```python
from build123d import *

# Parameters (mm, degrees)
SKETCH1_W           = 76.454
SKETCH1_H           = 69.596
BOSS_EXTRUDE1_DEPTH = 7.62
SKETCH2_W           = 71.374
SKETCH2_H           = 64.516
CUT_EXTRUDE1_DEPTH  = 5.08
SKETCH4_W           = 5.08
SKETCH4_H           = 5.08
BOSS_EXTRUDE2_DEPTH = 8.7884
CUT_EXTRUDE2_DEPTH  = 5.08
SKETCH6_W           = 2.54
SKETCH6_H           = 2.54
BOSS_EXTRUDE3_DEPTH = 29.21
SKETCH7_W           = 76.454
SKETCH7_H           = 69.596
BOSS_EXTRUDE4_DEPTH = 2.54
CUT_EXTRUDE3_REACH  = 50.158
SKETCH8_W           = 5.08
SKETCH8_H           = 5.08


with BuildPart() as part:
    # Sketch1 → Boss-Extrude1 (new body)
    with BuildSketch(Plane(origin=(0, 0, 0), x_dir=(1, 0, 0), z_dir=(0, 1, 0))):
        Rectangle(SKETCH1_W, SKETCH1_H)
    extrude(amount=-BOSS_EXTRUDE1_DEPTH)

    # Sketch2 → Cut-Extrude1 (cut)
    with BuildSketch(Plane(origin=(0, 0, 0), x_dir=(1, 0, 0), z_dir=(0, 1, 0))):
        Rectangle(SKETCH2_W, SKETCH2_H)
    extrude(amount=-CUT_EXTRUDE1_DEPTH, mode=Mode.SUBTRACT)

    # Sketch4 → Boss-Extrude2 (add)
    with BuildSketch(Plane.XZ.offset(7.62)):
        with Locations((-29.972, 26.543)):
            Rectangle(SKETCH4_W, SKETCH4_H)
        with Locations((29.972, 26.543)):
            Rectangle(SKETCH4_W, SKETCH4_H)
    boss_extrude2 = extrude(amount=BOSS_EXTRUDE2_DEPTH)

    # Sketch5 → Cut-Extrude2 (cut)
    with BuildSketch(Plane.XY.offset(29.083)):
        Polygon((29.972, -16.4084), (27.432, -12.606876095), (27.432, -16.4084), align=None)
        Polygon((-29.972, -16.4084), (-32.512, -12.606876095), (-32.512, -16.4084), align=None)
        Polygon((27.432, -11.336876095), (29.153074553, -10.798216701), (29.153074553, -7.62), (27.432, -7.62), align=None)
        Polygon((-32.512, -11.336876095), (-30.790925447, -10.798216701), (-30.790925447, -7.62), (-32.512, -7.62), align=None)
    cut_extrude2 = extrude(amount=-CUT_EXTRUDE2_DEPTH, mode=Mode.SUBTRACT)

    # Mirror1: Boss-Extrude2, Cut-Extrude2 across plane
    add(boss_extrude2.mirror(Plane.XY))
    add(cut_extrude2.mirror(Plane.XY), mode=Mode.SUBTRACT)

    # Sketch6 → Boss-Extrude3 (add)
    with BuildSketch(Plane(origin=(0, 0, 0), x_dir=(1, 0, 0), z_dir=(0, 1, 0))):
        with Locations((-36.957, 33.528)):
            Rectangle(SKETCH6_W, SKETCH6_H)
        with Locations((-36.957, -33.528)):
            Rectangle(SKETCH6_W, SKETCH6_H)
        with Locations((36.957, -33.528)):
            Rectangle(SKETCH6_W, SKETCH6_H)
        with Locations((36.957, 33.528)):
            Rectangle(SKETCH6_W, SKETCH6_H)
    extrude(amount=BOSS_EXTRUDE3_DEPTH)

    # Sketch7 → Boss-Extrude4 (add)
    with BuildSketch(Plane(origin=(0, 29.21, 0), x_dir=(1, 0, 0), z_dir=(0, 1, 0))):
        Rectangle(SKETCH7_W, SKETCH7_H)
    extrude(amount=BOSS_EXTRUDE4_DEPTH)

    # Sketch8 → Cut-Extrude3 (cut, up to next)
    with BuildSketch(Plane(origin=(0, 31.75, 0), x_dir=(1, 0, 0), z_dir=(0, 1, 0)), mode=Mode.PRIVATE) as cut_extrude3_sk1:
        with Locations((29.845, 20.8788)):
            Rectangle(SKETCH8_W, SKETCH8_H)
    cut_extrude3_tool1 = extrude(cut_extrude3_sk1.sketch, amount=-CUT_EXTRUDE3_REACH, mode=Mode.PRIVATE) & part.part
    add(cut_extrude3_tool1.solids().sort_by_distance((29.845, 31.75, -20.8788))[0], mode=Mode.SUBTRACT)
    # Sketch8 → Cut-Extrude3 (cut, up to next)
    with BuildSketch(Plane(origin=(0, 31.75, 0), x_dir=(1, 0, 0), z_dir=(0, 1, 0)), mode=Mode.PRIVATE) as cut_extrude3_sk2:
        with Locations((-29.845, 20.8788)):
            Rectangle(SKETCH8_W, SKETCH8_H)
    cut_extrude3_tool2 = extrude(cut_extrude3_sk2.sketch, amount=-CUT_EXTRUDE3_REACH, mode=Mode.PRIVATE) & part.part
    add(cut_extrude3_tool2.solids().sort_by_distance((-29.845, 31.75, -20.8788))[0], mode=Mode.SUBTRACT)
    # Sketch8 → Cut-Extrude3 (cut, up to next)
    with BuildSketch(Plane(origin=(0, 31.75, 0), x_dir=(1, 0, 0), z_dir=(0, 1, 0)), mode=Mode.PRIVATE) as cut_extrude3_sk3:
        with Locations((29.845, -20.8788)):
            Rectangle(SKETCH8_W, SKETCH8_H)
    cut_extrude3_tool3 = extrude(cut_extrude3_sk3.sketch, amount=-CUT_EXTRUDE3_REACH, mode=Mode.PRIVATE) & part.part
    add(cut_extrude3_tool3.solids().sort_by_distance((29.845, 31.75, 20.8788))[0], mode=Mode.SUBTRACT)
    # Sketch8 → Cut-Extrude3 (cut, up to next)
    with BuildSketch(Plane(origin=(0, 31.75, 0), x_dir=(1, 0, 0), z_dir=(0, 1, 0)), mode=Mode.PRIVATE) as cut_extrude3_sk4:
        with Locations((-29.845, -20.8788)):
            Rectangle(SKETCH8_W, SKETCH8_H)
    cut_extrude3_tool4 = extrude(cut_extrude3_sk4.sketch, amount=-CUT_EXTRUDE3_REACH, mode=Mode.PRIVATE) & part.part
    add(cut_extrude3_tool4.solids().sort_by_distance((-29.845, 31.75, 20.8788))[0], mode=Mode.SUBTRACT)


solid = part.part
```
Could you check a few things on this model? Use its own coordinates, in mm. A direction names the side the tool comes from. Coordinates: 2 decimals unless noted, no trailing zeros. Write each loop counter-clockwise with the first axis right and the second up, starting at its lowest first coordinate (ties: lowest second). Pieces come first, ordered by that corner, then holes. Notation, with made-up numbers: (42.5, -31) -> (68.5, -31) arc R22 ccw to (68.5, 3) -> close; hole circle Ø6 at (11, 38.25). An arc over 180 degrees is marked (long way). One line per question, with ' | ' between items. Start each with the question number.
1. Will these pins go through, and if not, where does the flat tip stop? P1, Ø2.5, axis at y = -13, z = -27.5, coming from the +X side; P2, Ø1.4, axis at y = -11.5, z = -27.5, coming from the -X side; P3, Ø1, axis at x = 27.5, z = -26, coming from the -Y side.
2. Thinking about a two-plate mould opening in Y: for faces 1 (the face through (-27.432, -12, -27)), 2 (the face through (-35.687, 14, -34)), which applies, pulls with the +Y half, pulls with the -Y half, needs draft (parallel to the pull), parting line crosses it, or undercut?
3. If we section it at C-C (z = -9): Please give me the cut outline in (x, y).
4. For faces 3 (the face through (32.512, -12, -27)), 4 (the face through (37, 14, 32.258)), 5 (the face through (-29, -12, -24.003)), which set-ups out of +Z, -Z, +X, -X, +Y, -Y let a thin tool reach every point of the face, with its end or its side?
5. If we section it at B-B (x = -4.5): Please give me the cut outline in (y, z), and give its area (3 significant figures).
6. If we section it at D-D (z = 22): Please give me the cut outline in (x, y) (3 decimals).
7. Please list where these lines run through material, in increasing order: line 1 along Z through (x, y) = (31, -4.5); line 2 along Y through (x, z) = (32, 29); line 3 along Y through (x, z) = (29, -30.5).
8. If we section it at A-A (y = 13): Please give me the cut outline in (x, z).
Return value:
1) P1: stops at x = 32.51 | P2: stops at x = -32.51 | P3: stops at y = -13.46
2) face 1: needs draft | face 2: undercut
3) outline: (-38.23, -7.62) -> (38.23, -7.62) -> (38.23, 0) -> (35.69, 0) -> (35.69, -5.08) -> (-35.69, -5.08) -> (-35.69, 0) -> (-38.23, 0) -> close; (-38.23, 29.21) -> (38.23, 29.21) -> (38.23, 31.75) -> (-38.23, 31.75) -> close
4) face 3: +Z, -Z, +X, -Y | face 4: +X, -X | face 5: +X, -X, -Y
5) outline: (-7.62, -34.8) -> (0, -34.8) -> (0, -32.26) -> (-5.08, -32.26) -> (-5.08, 32.26) -> (0, 32.26) -> (0, 34.8) -> (-7.62, 34.8) -> close; (29.21, -34.8) -> (31.75, -34.8) -> (31.75, 34.8) -> (29.21, 34.8) -> close | area: 379 mm²
6) outline: (-38.227, -7.62) -> (38.227, -7.62) -> (38.227, 0) -> (35.687, 0) -> (35.687, -5.08) -> (-35.687, -5.08) -> (-35.687, 0) -> (-38.227, 0) -> close; (-38.227, 29.21) -> (-32.385, 29.21) -> (-32.385, 31.75) -> (-38.227, 31.75) -> close; (-27.305, 29.21) -> (27.305, 29.21) -> (27.305, 31.75) -> (-27.305, 31.75) -> close; (32.385, 29.21) -> (38.227, 29.21) -> (38.227, 31.75) -> (32.385, 31.75) -> close
7) line 1: z = -34.8 to -32.26, 32.26 to 34.8 | line 2: y = -16.41 to -5.08, 29.21 to 31.75 | line 3: y = -7.62 to -5.08, 29.21 to 31.75
8) outline: (-38.23, -34.8) -> (-35.69, -34.8) -> (-35.69, -32.26) -> (-38.23, -32.26) -> close; (-38.23, 32.26) -> (-35.69, 32.26) -> (-35.69, 34.8) -> (-38.23, 34.8) -> close; (35.69, -34.8) -> (38.23, -34.8) -> (38.23, -32.26) -> (35.69, -32.26) -> close; (35.69, 32.26) -> (38.23, 32.26) -> (38.23, 34.8) -> (35.69, 34.8) -> close
